```python
from build123d import *
from build123d.topology import SkipClean

# Parameters (mm, degrees)
SKETCH1_R               = 20
SKETCH1_R_2             = 19
BOSS_EXTRUDE1_DEPTH     = 22
FILLET1_R               = 0.5
SKETCH5_W               = 9
SKETCH5_H               = 1
CUT_EXTRUDE1_DEPTH      = 10
CUT_EXTRUDE1_DEPTH_BACK = 10
SKETCH6_R               = 14.25
BOSS_EXTRUDE2_START     = -44
BOSS_EXTRUDE2_DEPTH     = 4
CHAMFER1_SIZE           = 1


with BuildPart() as part:
    # Sketch1 → Boss-Extrude1 (new body)
    with BuildSketch(Plane.XY):
        Circle(SKETCH1_R)
        Circle(SKETCH1_R_2, mode=Mode.SUBTRACT)
    extrude(amount=BOSS_EXTRUDE1_DEPTH)

    # Fillet1
    fillet1_edges = [part.edges().sort_by_distance(p)[0] for p in [
        (-20, 0, 22),
    ]]
    fillet(fillet1_edges, radius=FILLET1_R)

    # Sketch5 → Revolve1 (revolve)
    with BuildSketch(Plane(origin=(0, 0, 0), x_dir=(0, 0, -1), z_dir=(1, 0, 0)), mode=Mode.PRIVATE) as revolve1_sk:
        Polygon((0, 19), (18, 6), (18, 7), (0, 20), align=None)
        with Locations((22.5, 6.5)):
            Rectangle(SKETCH5_W, SKETCH5_H)
    revolve(revolve1_sk.sketch.rotate(Axis((0, 0, 0), (0, 0, -1)), 90), axis=Axis((0, 0, 0), (0, 0, -1)))

    # Sketch6 → Cut-Extrude1 (cut, two sides: drawn at the far end of the back side and taken through both)
    with BuildSketch(Plane(origin=(0, 0, 0), x_dir=(0, 0, -1), z_dir=(1, 0, 0)).offset(-CUT_EXTRUDE1_DEPTH_BACK)):
        with Locations((39.412191587, 0)):
            Circle(SKETCH6_R)
    extrude(amount=CUT_EXTRUDE1_DEPTH + CUT_EXTRUDE1_DEPTH_BACK, mode=Mode.SUBTRACT)

    # Sketch7 → Boss-Extrude2 (add)
    with SkipClean():  # the faces are left unmerged after this step: merging them gives an invalid solid
        with BuildSketch(Plane.XY.offset(22).offset(BOSS_EXTRUDE2_START)):
            with BuildLine():
                Line((-6.92820323, -1), (-5, -1))
                Line((-5, -1), (-5, 1))
                Line((-5, 1), (-6.92820323, 1))
                ThreePointArc((-6.92820323, 1), (-6.982027736, 0.501287038), (-7, 0))
                ThreePointArc((-7, 0), (-6.982027736, -0.501287038), (-6.92820323, -1))
            make_face()
            with BuildLine():
                Line((5, -1), (6.92820323, -1))
                ThreePointArc((6.92820323, -1), (6.982027736, -0.501287038), (7, 0))
                ThreePointArc((7, 0), (6.982027736, 0.501287038), (6.92820323, 1))
                Line((6.92820323, 1), (5, 1))
                Line((5, 1), (5, -1))
            make_face()
        extrude(amount=BOSS_EXTRUDE2_DEPTH)

    # Chamfer1
    chamfer1_edges = [part.edges().sort_by_distance(p)[0] for p in [
        (-5, 0, -22),
        (5, 0, -22),
    ]]
    chamfer(chamfer1_edges, length=CHAMFER1_SIZE - 0.0001)  # a hair under: the kernel refuses the full size


solid = part.part
```
Input: part model. Units: mm. Frame: model coordinates. A direction names the side the tool comes from. Give positions to 0.01 mm unless a question says otherwise; leave off trailing zeros. Write each loop counter-clockwise with the first axis right and the second up, starting at its lowest first coordinate (ties: lowest second). Pieces come first, ordered by that corner, then holes. Notation, with made-up numbers: (-4, -5) - (53, -5) arc R26 cw to (53, 12) - close; hole circle Ø10 at (61, 84.5). An arc over 180 degrees is marked (long way). Write item = value, one per line. Start each with the question number.
1. Ray query, L1, parallel to Y at x = 0, z = -23; L2, parallel to Y at x = 0, z = 13.75; L3, parallel to X at y = 4.5, z = 4.5. Return the intervals inside material, ascending.
2. Section query A-A, the plane x = 0. Output: boundary loops of the cut face in (y, z), then the cut area to 3 significant figures.
3. First-contact query: pin 1 Ø0.5 at (x, z) = (5.5, -19.5) entering from -Y; pin 2 Ø3 at (x, y) = (13, -1) entering from -Z; pin 3 Ø10 at (y, z) = (9.5, -12) entering from -X. Flat tips, straight axial feed; report the tip coordinate or a pass-through.
4. Mould query, pull axis Y, two halves, no side actions, for faces 4 (the cylindrical face through (-5.555, 4.259, -22.563)), 5 (the flat face through (4.2, -18.7, 22)), 6 (the cylindrical face through (3.078, 5.323, -26.194)), 7 (the flat face through (-5, 0, -20)). Classes: released by +Y, released by -Y, zero draft, split by the parting line, or undercut.
5. Section query B-B, the plane z = 19. Output: boundary loops of the cut face in (x, y), then the cut area to 3 significant figures.
6. Access query for faces 1 (the conical face through (8.83, -2.781, -14.874)), 2 (the cylindrical face through (8.767, -16.856, 10.846)), 3 (the flat face through (5, 0, -20)). Directions: +Z, -Z, +X, -X, +Y, -Y. A direction counts if a zero-diameter tool reaches every point of the face in a straight line with its end or side. Return the directions, or none.
Check sheet entries:
q1.L1 = -7 to -6, 6 to 7
q1.L2 = -20 to -19, 19 to 20
q1.L3 = -19.49 to -18.46, 18.46 to 19.49
q2.outline = (-20, 0) - (-7, -18) - (-7, -27) arc R14.25 cw to (-6, -26.49) - (-6, -18) - (-19, 0) - (-19, 22) - (-19.5, 22) arc R0.5 ccw to (-20, 21.5) - close; (6, -26.49) arc R14.25 cw to (7, -27) - (7, -18) - (20, 0) - (20, 21.5) arc R0.5 ccw to (19.5, 22) - (19, 22) - (19, 0) - (6, -18) - close
q2.area = 97.4 mm2
q3.pin_1 = -4.63
q3.pin_2 = -11.72
q3.pin_3 = -12.66
q4.face_4 = split by the parting line
q4.face_5 = zero draft
q4.face_6 = undercut
q4.face_7 = undercut
q5.outline = circle Ø40 at (0, 0); hole circle Ø38 at (0, 0)
q5.area = 123 mm2
q6.face_1 = -Z
q6.face_2 = +Z
q6.face_3 = +Z, -Z
